Verification items for the finished model (mm, model axes). Face numbers are marked on the shaded views. A direction names the side the tool comes from. Coordinates: 2 decimals unless noted, no trailing zeros. Order: outer loops, then holes, each group sorted by start corner. A loop starts at its lowest first (then second) coordinate and runs counter-clockwise, first axis right, second up. Notation, with made-up numbers: M 2,40 L 38,40 A11 ccw 38,51 Z; hole C 70,89 d8. An arc over 180 degrees is marked long. Answer as a JSON object with one key per item and string values. Group by question number.
(1) Cross-section at C-C (x = -9.5). Enter the section's corners in (y, z), plus the area to 4 significant figures.
(2) Material ranges on line 1 (X direction, y = -1.5, z = 9.5), recorded low to high.
(3) Gauge pin test, flat end, axial feed: pin 1 Ø3 at (x, y) = (1.5, -4.5) entering from +Z. Record the tip position at first contact, or that the pin passes through.
(4) Cross-section at A-A (z = 6). Enter the section's corners in (x, y), plus the area to 4 significant figures.
(5) Mould release check, pull along Y, two halves, no side actions. Record for the marked faces 1, 2 and 3: released by +Y, released by -Y, zero draft, split by the parting line, or undercut.
(6) Access from +Z, -Z, +X, -X, +Y, -Y to the whole of each face (thin tool, end or side, straight path). Record for the marked faces 4, 5, 6, 7 and 8.
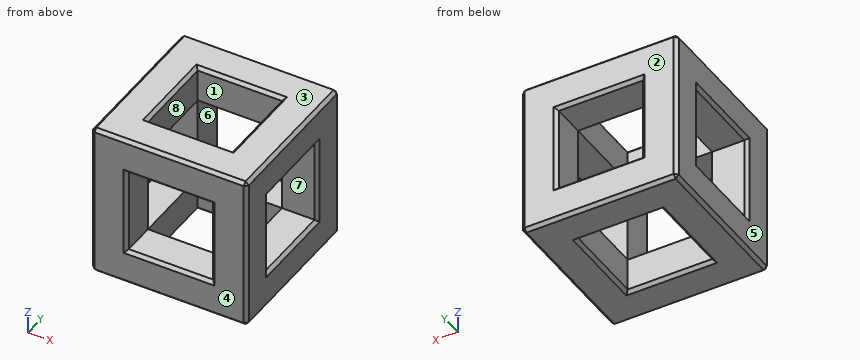
from build123d import *

# Parameters (mm, degrees)
F0_W          = 24
F0_H          = 24
F0_W_2        = 13
F0_H_2        = 13
F1_DEPTH      = 12
F1_DEPTH_BACK = 12
F2_W          = 13
F2_H          = 13
F3_DEPTH      = 24.001
F4_W          = 13
F4_H          = 13
F5_DEPTH      = 24.001
F6_SIZE       = 0.5


with BuildPart() as f1:
    # F0 (on Top) → F1 (new body, two sides)
    with BuildSketch(Plane.XY) as f1_sk:
        Rectangle(F0_W, F0_H)
        Rectangle(F0_W_2, F0_H_2, mode=Mode.SUBTRACT)
    extrude(amount=F1_DEPTH)
    extrude(f1_sk.sketch, amount=-F1_DEPTH_BACK)

    # F2 (on face) → F3 (cut, through all)
    with BuildSketch(Plane.XZ.offset(12)):
        Rectangle(F2_W, F2_H)
    extrude(amount=-F3_DEPTH, mode=Mode.SUBTRACT)

    # F4 (on face) → F5 (cut, through all)
    with BuildSketch(Plane.YZ.offset(12)):
        Rectangle(F4_W, F4_H)
    extrude(amount=-F5_DEPTH, mode=Mode.SUBTRACT)

    # F6
    f6_edges = [f1.edges().sort_by_distance(p)[0] for p in [
        (-12, 0, 12),
        (-12, 12, 0),
        (-12, 0, -12),
        (-12, -12, 0),
        (12, 0, 12),
        (12, 12, 0),
        (12, 0, -12),
        (12, -12, 0),
        (0, 12, -12),
        (0, 12, 12),
        (0, -12, -12),
        (0, -12, 12),
        (6.5, 0, 12),
        (0, 6.5, 12),
        (-6.5, 0, 12),
        (0, -6.5, 12),
        (6.5, -12, 0),
        (0, -12, 6.5),
        (-6.5, -12, 0),
        (0, -12, -6.5),
        (12, -6.5, 0),
        (12, 0, 6.5),
        (12, 6.5, 0),
        (12, 0, -6.5),
        (6.5, 12, 0),
        (0, 12, 6.5),
        (-6.5, 12, 0),
        (0, 12, -6.5),
        (0, 6.5, -12),
        (6.5, 0, -12),
        (0, -6.5, -12),
        (-6.5, 0, -12),
        (-12, 0, -6.5),
        (-12, 6.5, 0),
        (-12, 0, 6.5),
        (-12, -6.5, 0),
    ]]
    chamfer(f6_edges, length=F6_SIZE)


solid = f1.part
Taken from the geometry:
{
 "1": {"outline": "M -12,-11.5 L -11.5,-12 L 11.5,-12 L 12,-11.5 L 12,11.5 L 11.5,12 L -11.5,12 L -12,11.5 Z; hole M -6.5,-6.5 L 6.5,-6.5 L 6.5,6.5 L -6.5,6.5 Z", "area": "406.5 mm²"},
 "2": {"line 1": "x = -12 to -6.5, 6.5 to 12"},
 "3": {"pin 1": "passes through"},
 "4": {"outline": "M -12,-11.5 L -11.5,-12 L -7,-12 L -6.5,-11.5 L -6.5,-6.5 L -11.5,-6.5 L -12,-7 Z; M -12,7 L -11.5,6.5 L -6.5,6.5 L -6.5,11.5 L -7,12 L -11.5,12 L -12,11.5 Z; M 6.5,-11.5 L 7,-12 L 11.5,-12 L 12,-11.5 L 12,-7 L 11.5,-6.5 L 6.5,-6.5 Z; M 6.5,6.5 L 11.5,6.5 L 12,7 L 12,11.5 L 11.5,12 L 7,12 L 6.5,11.5 Z", "area": "119.5 mm²"},
 "5": {"face 1": "undercut", "face 2": "released by +Y", "face 3": "zero draft"},
 "6": {"face 4": "+Z, -Z, +X, -X, -Y", "face 5": "+Z, -Z, -X, +Y, -Y", "face 6": "+Y, -Y", "face 7": "+X, -X", "face 8": "+Z, -Z"}
}
